Geometry check sheet. Reference: the model listing, model coordinates, mm. Give positions to 0.01 mm unless a question says otherwise; leave off trailing zeros. Loops run counter-clockwise (first coordinate to the right, second up) from the corner with the lowest first, then second, coordinate; pieces in that order, holes last.
```python
from build123d import *

# Parameters (mm, degrees)
EXTRUDE1_DEPTH     = 5.5
SKETCH2_R          = 1.5
SKETCH2_R_2        = 1.25
CUT_EXTRUDE1_DEPTH = 22.5


with BuildPart() as part:
    # Sketch1 → Extrude1 (new body, symmetric)
    with BuildSketch(Plane.XY):
        with BuildLine():
            Line((-164.827821897, 11.989846995), (-255.561088457, 2.5))
            Line((-255.561088457, 2.5), (-274.839724553, 2.5))
            Line((-274.839724553, 2.5), (-274.839724553, 3.5))
            Line((-274.839724553, 3.5), (-165.139891452, 14.973571613))
            ThreePointArc((-165.139891452, 14.973571613), (-102.654981247, 19.86728494), (-40, 21.5))
            Line((-40, 21.5), (0, 21.5))
            Line((0, 21.5), (0, 18.5))
            Line((0, 18.5), (-40, 18.5))
            ThreePointArc((-40, 18.5), (-102.498734411, 16.871356549), (-164.827821897, 11.989846995))
        make_face()
    extrude(amount=EXTRUDE1_DEPTH, both=True)

    # Sketch2 → Cut-Extrude1 (cut, through all)
    with BuildSketch(Plane(origin=(0, 0, 0), x_dir=(1, 0, 0), z_dir=(0, 1, 0))):
        with Locations(Location((-63, 0, 0), (0, 0, 90))):  # turned: the seam where the file's is
            Circle(SKETCH2_R)
        with Locations(Location((-78, 0, 0), (0, 0, 90))):  # turned: the seam where the file's is
            Circle(SKETCH2_R_2)
    extrude(amount=CUT_EXTRUDE1_DEPTH, mode=Mode.SUBTRACT)


solid = part.part
```
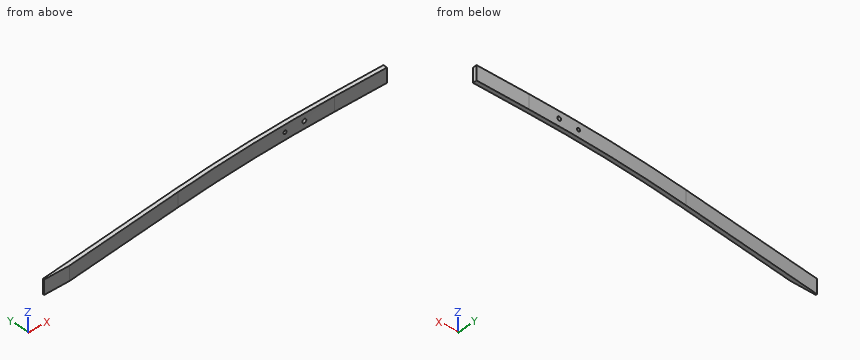
1) Scan lines: line 1 along Z through (x, y) = (-78, 18.85); line 2 along Y through (x, z) = (-22, 1.5); line 3 along Y through (x, z) = (-63.5, 5.25). Record each from-to range of solid material in increasing order.
2) Sectioned sample at A-A on z = -3.25. Enter the section's corners in (x, y).
3) Sectioned sample at B-B on x = -21. Enter the section's corners in (y, z), plus the area to 3 significant figures.
4) Sectioned sample at C-C on x = -241. Enter the section's corners in (y, z), plus the area to 3 significant figures.
5) Depth check by flat-ended pin: P1, Ø2, axis at x = -78, z = 0, coming from the +Y side; P2, Ø3.5, axis at x = -63, z = 0, coming from the -Y side; P3, Ø1, axis at x = -139, z = -1.5, coming from the -Y side. Enter the tip coordinate at first touch or a pass-through.
Determined:
1. line 1: z = -5.5 to -1.25, 1.25 to 5.5
1. line 2: y = 18.5 to 21.5
1. line 3: y = 18.27 to 21.27
2. outline: (-274.84, 2.5) - (-255.56, 2.5) - (-164.83, 11.99) arc R1200 cw to (-40, 18.5) - (0, 18.5) - (0, 21.5) - (-40, 21.5) arc R1203 ccw to (-165.14, 14.97) - (-274.84, 3.5) - close
3. outline: (18.5, -5.5) - (21.5, -5.5) - (21.5, 5.5) - (18.5, 5.5) - close
3. area: 33.0 mm2
4. outline: (4.02, -5.5) - (7.04, -5.5) - (7.04, 5.5) - (4.02, 5.5) - close
4. area: 33.2 mm2
5. P1: passes through
5. P2: stops at y = 18.24
5. P3: stops at y = 14.37
